Geometry check sheet. Reference: the model listing, model coordinates, mm. A direction names the side the tool comes from. Coordinates: 2 decimals unless noted, no trailing zeros. Write each loop counter-clockwise with the first axis right and the second up, starting at its lowest first coordinate (ties: lowest second). Pieces come first, ordered by that corner, then holes. Notation, with made-up numbers: (-21.5, 33.25) -> (23.5, 33.25) arc R22 ccw to (23.5, 48.25) -> close; hole circle Ø3 at (26, 82.5). An arc over 180 degrees is marked (long way). Use a Markdown table: item, result.
```python
from build123d import *

# Parameters (mm, degrees)
CROQUIS1_R              = 2
CROQUIS1_R_2            = 2.5
CROQUIS1_R_3            = 1.5
SALIENTE_EXTRUIR1_DEPTH = 3


with BuildPart() as part:
    # Croquis1 → Saliente-Extruir1 (new body)
    with BuildSketch(Plane.XY):
        with BuildLine():
            Line((1.762553306, 0), (-1.762553306, 0))
            ThreePointArc((-1.762553306, 0), (-3.476899283, 0.538086543), (-4.576267594, 1.95932142))
            Line((-4.576267594, 1.95932142), (-14.815986324, 29.644759985))
            ThreePointArc((-14.815986324, 29.644759985), (-14.464185493, 32.399784542), (-12.002272036, 33.685438565))
            Line((-12.002272036, 33.685438565), (-10.5, 33.685438565))
            Line((-10.5, 33.685438565), (-10.5, 133))
            ThreePointArc((-10.5, 133), (-10.856456095, 134.854049622), (-11.875, 136.443744328))
            ThreePointArc((-11.875, 136.443744328), (-14.930631716, 141.212828449), (-16, 146.774977314))
            Line((-16, 146.774977314), (-16, 155))
            ThreePointArc((-16, 155), (-11.606601718, 165.606601718), (-1, 170))
            Line((-1, 170), (1, 170))
            ThreePointArc((1, 170), (11.606601718, 165.606601718), (16, 155))
            Line((16, 155), (16, 146.774977314))
            ThreePointArc((16, 146.774977314), (14.930631716, 141.212828449), (11.875, 136.443744328))
            ThreePointArc((11.875, 136.443744328), (10.856456095, 134.854049622), (10.5, 133))
            Line((10.5, 133), (10.5, 33.685438565))
            Line((10.5, 33.685438565), (12.002272036, 33.685438565))
            ThreePointArc((12.002272036, 33.685438565), (14.464185493, 32.399784542), (14.815986324, 29.644759985))
            Line((14.815986324, 29.644759985), (4.576267594, 1.95932142))
            ThreePointArc((4.576267594, 1.95932142), (3.476899283, 0.538086543), (1.762553306, 0))
        make_face()
        with Locations((0, 6)):
            Circle(CROQUIS1_R, mode=Mode.SUBTRACT)
        with Locations((0, 150.5)):
            Circle(CROQUIS1_R_2, mode=Mode.SUBTRACT)
        with Locations((0, 144.5)):
            Circle(CROQUIS1_R_3, mode=Mode.SUBTRACT)
        with Locations((-6, 150.5)):
            Circle(CROQUIS1_R_3, mode=Mode.SUBTRACT)
        with Locations(Location((0, 156.5, 0), (0, 0, 180))):
            Circle(CROQUIS1_R_3, mode=Mode.SUBTRACT)
        with Locations(Location((6, 150.5, 0), (0, 0, 180))):
            Circle(CROQUIS1_R_3, mode=Mode.SUBTRACT)
        with Locations((-8, 29.685438565)):
            Circle(CROQUIS1_R, mode=Mode.SUBTRACT)
        with Locations((8, 29.685438565)):
            Circle(CROQUIS1_R, mode=Mode.SUBTRACT)
        with Locations((0, 15.55)):
            Circle(CROQUIS1_R, mode=Mode.SUBTRACT)
    extrude(amount=SALIENTE_EXTRUIR1_DEPTH)


solid = part.part
```
Item 1: Depth check by flat-ended pin: P1, Ø0.5, axis at x = 11, z = 2, coming from the +Y side; P2, Ø0.9, axis at y = 82.5, z = 1.5, coming from the +X side; P3, Ø3.5, axis at x = 8, y = 29.69, coming from the -Z side; P4, Ø0.8, axis at x = -11, z = 1.5, coming from the +Y side. Enter the tip coordinate at first touch or a pass-through.
Answer block:
| item | result |
|---|---|
| P1 | stops at y = 166.4 |
| P2 | stops at x = 10.5 |
| P3 | passes through |
| P4 | stops at y = 166.53 |
Item 2: Section check C-C on y = 78. Record the boundary of the cut face in (x, z), then the cut area to 3 significant figures.
Answer block:
| item | result |
|---|---|
| outline | (-10.5, 0) -> (10.5, 0) -> (10.5, 3) -> (-10.5, 3) -> close |
| area | 63.0 mm^2 |
Item 3: Section check D-D on y = 144.5. Record the boundary of the cut face in (x, z), then the cut area to 3 significant figures.
Answer block:
| item | result |
|---|---|
| outline | (-15.83, 0) -> (-1.5, 0) -> (-1.5, 3) -> (-15.83, 3) -> close; (1.5, 0) -> (15.83, 0) -> (15.83, 3) -> (1.5, 3) -> close |
| area | 86.0 mm^2 |
Item 4: Mould release check, pull along Y, two halves, no side actions. Record for faces 4 (the flat face through (0, 0, 1)), 5 (the cylindrical face through (-6, 152, 1)), 6 (the flat face through (16, 151, 1)): +Y half, -Y half, draft (parallel to the pull), parting line (faces both ways), or undercut.
Answer block:
| item | result |
|---|---|
| face 4 | -Y half |
| face 5 | undercut |
| face 6 | draft |
Item 5: Tool access check on faces 1 (the cylindrical face through (0, 155, 1)), 2 (the cylindrical face through (10.866, 134.879, 1.479)), 3 (the cylindrical face through (-10.847, 134.829, 1.479)). Record the directions out of +Z, -Z, +X, -X, +Y, -Y that give a thin tool (end or side, any length) a straight path to the whole face; none if there is none.
Answer block:
| item | result |
|---|---|
| face 1 | +Z, -Z |
| face 2 | +Z, -Z, +X |
| face 3 | +Z, -Z, -X |
Item 6: Thickness scan on L1, parallel to Y at x = 0, z = 1.55; L2, parallel to X at y = 150.5, z = 0.75; L3, parallel to X at y = 118.5, z = 0.55. Record the ranges inside material, lowest first. Write a range as [from, to].
Answer block:
| item | result |
|---|---|
| L1 | y = [0, 4], [8, 13.55], [17.55, 143], [146, 148], [153, 155], [158, 170] |
| L2 | x = [-16, -7.5], [-4.5, -2.5], [2.5, 4.5], [7.5, 16] |
| L3 | x = [-10.5, 10.5] |
Item 7: Section check A-A on z = 2.5. Count the separate pieces of the cut face and the enclosed holes in it, then the cut area to 3 significant figures.
Answer block:
| item | result |
|---|---|
| separate pieces | 1 |
| enclosed holes | 9 |
| area | 3,680 mm^2 |
Item 8: Section check B-B on y = 6. Record the boundary of the cut face in (x, z), then the cut area to 3 significant figures.
Answer block:
| item | result |
|---|---|
| outline | (-6.07, 0) -> (-2, 0) -> (-2, 3) -> (-6.07, 3) -> close; (2, 0) -> (6.07, 0) -> (6.07, 3) -> (2, 3) -> close |
| area | 24.4 mm^2 |
